from build123d import *

# Parameters (mm, degrees)
SKETCH1_R           = 5
BOSS_EXTRUDE1_DEPTH = 7
FILLET1_R           = 5
BOSS_EXTRU_1_DEPTH  = 0.5


with BuildPart() as part:
    # Sketch1 → Boss-Extrude1 (new body)
    with BuildSketch(Plane(origin=(0, 0, 0), x_dir=(1, 0, 0), z_dir=(0, 1, 0))):
        Circle(SKETCH1_R)
    extrude(amount=BOSS_EXTRUDE1_DEPTH)

    # Fillet1
    fillet1_edges = [part.edges().sort_by_distance(p)[0] for p in [
        (-5, 7, 0),
    ]]
    fillet(fillet1_edges, radius=FILLET1_R)

    # Esquisse1 → Boss.-Extru.1 (add)
    with BuildSketch(Plane.XZ):
        with BuildLine():
            Line((-2.5, 8), (-2.5, 4.330127019))
            ThreePointArc((-2.5, 4.330127019), (0, 5), (2.5, 4.330127019))
            Line((2.5, 4.330127019), (2.5, 8))
            ThreePointArc((2.5, 8), (0, 10.5), (-2.5, 8))
        make_face()
        with BuildLine():
            ThreePointArc((-4.330127019, -2.5), (-5, 0), (-4.330127019, 2.5))
            Line((-4.330127019, 2.5), (-8, 2.5))
            ThreePointArc((-8, 2.5), (-10.5, 0), (-8, -2.5))
            Line((-8, -2.5), (-4.330127019, -2.5))
        make_face()
        with BuildLine():
            Line((8, 2.5), (4.330127019, 2.5))
            ThreePointArc((4.330127019, 2.5), (5, 0), (4.330127019, -2.5))
            Line((4.330127019, -2.5), (8, -2.5))
            ThreePointArc((8, -2.5), (10.5, 0), (8, 2.5))
        make_face()
        with BuildLine():
            ThreePointArc((2.5, -4.330127019), (0, -5), (-2.5, -4.330127019))
            Line((-2.5, -4.330127019), (-2.5, -8))
            ThreePointArc((-2.5, -8), (0, -10.5), (2.5, -8))
            Line((2.5, -8), (2.5, -4.330127019))
        make_face()
    extrude(amount=-BOSS_EXTRU_1_DEPTH)


solid = part.part
For this review, take the finished solid that the model builds, in its own axes (mm). A direction names the side the tool comes from. Give positions to 0.01 mm unless a question says otherwise; leave off trailing zeros. Loops run counter-clockwise (first coordinate to the right, second up) from the corner with the lowest first, then second, coordinate; pieces in that order, holes last.
Item 1: Tool access review of faces 1 (the cylindrical face through (0.1, 0.2, 10.5)), 2 (the cylindrical face through (-4, 1, -3)): name each direction out of +Z, -Z, +X, -X, +Y, -Y from which nothing blocks a thin tool from reaching the whole face with its end or side.
Item 2: Take a section at A-A, the plane x = 0. State the section outline as (y, z) points, and give its area (3 significant figures).
Item 3: Insertion check: pin 1 (1.5 mm diameter, centred on x = -8.5, z = 0, fed in from +Y); pin 2 (5.5 mm diameter, centred on x = 0.5, z = -7, fed in from +Y); pin 3 (1.5 mm diameter, centred on y = 1, z = 7, fed in from +X). Each pin has a flat end and moves straight along its axis. Give the tip position at first contact, or say it passes through.
Item 4: Take a section at B-B, the plane z = 0. State the section outline as (x, y) points, and give its area (3 significant figures).
Item 5: Take a section at C-C, the plane y = 6. State the section outline as (x, z) points.
Item 6: For line 1 along Y through (x, z) = (5, -2); line 2 along Z through (x, y) = (-0.25, 1.75); line 3 along X through (y, z) = (2, 2.75), list the stretches that pass through material, from the lowest coordinate up.
Item 7: Take a section at D-D, the plane z = 6. State the section outline as (x, y) points, and give its area (3 significant figures).
Calculated:
1. face 1: +Z, +Y, -Y
1. face 2: +Y
2. outline: (0, -10.5) - (0.5, -10.5) - (0.5, -5) - (2, -5) arc R5 ccw to (2, 5) - (0.5, 5) - (0.5, 10.5) - (0, 10.5) - close
2. area: 64.8 mm2
3. pin 1: stops at y = 0.5
3. pin 2: stops at y = 4.6
3. pin 3: stops at x = 2.5
4. outline: (-10.5, 0) - (10.5, 0) - (10.5, 0.5) - (5, 0.5) - (5, 2) arc R5 ccw to (-5, 2) - (-5, 0.5) - (-10.5, 0.5) - close
4. area: 64.8 mm2
5. outline: circle Ø6 at (0, 0)
6. line 1: y = 0 to 0.5
6. line 2: z = -4.99 to 4.99
6. line 3: x = -4.18 to 4.18
7. outline: (-2.5, 0) - (2.5, 0) - (2.5, 0.5) - (-2.5, 0.5) - close
7. area: 2.50 mm2
